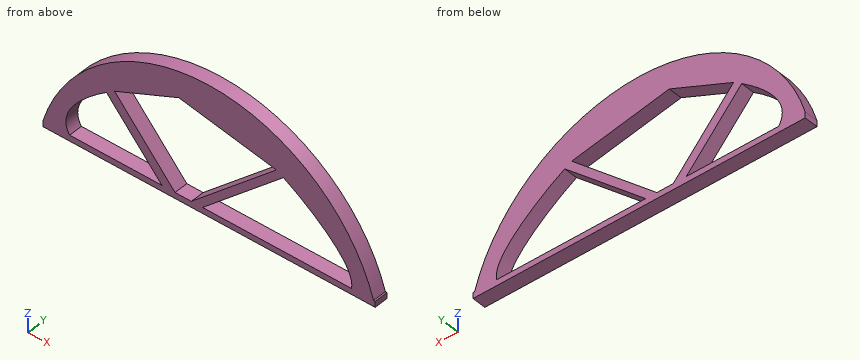
```python
from build123d import *

# Parameters (mm, degrees)
F1_DEPTH = 76.2


with BuildPart() as f1:
    # F0 (on Front) → F1 (new body)
    with BuildSketch(Plane.XZ):
        with BuildLine():
            Line((900.6498717056, -312.5507702395), (891.7103917568, -312.5507702395))
            ThreePointArc((891.7103917568, -312.5507702395), (-18.2198682688, 368.2339185386), (-928.1501282944, -312.5507702395))
            Line((-928.1501282944, -312.5507702395), (-928.1501282944, -345.05851352))
            Line((-928.1501282944, -345.05851352), (-749.2538985146, -345.05851352))
            add(Edge.make_bspline(
                [(-749.2538985146, -345.0585135201), (-760.7342074403, -336.2080146902), (-770.4190479747, -326.955384148), (-778.1336966335, -317.3006312947)],
                knots=[0.9863041687, 0.9863041687, 0.9863041687, 0.9863041687, 1, 1, 1, 1], degree=3))
            add(Edge.make_bspline(
                [(-778.1336966335, -317.3006312947), (-779.3903781429, -315.7279155528), (-780.5947807249, -314.1445295186), (-781.7476175602, -312.5507702395)],
                knots=[0, 0, 0, 0, 0.0022309892, 0.0022309892, 0.0022309892, 0.0022309892], degree=3))
            add(Edge.make_bspline(
                [(-781.7476175602, -312.5507702395), (-852.1024790666, -215.2874716318), (-730.4075461351, -79.390396257), (-578.7611195863, 27.6247892302)],
                knots=[0.0022309892, 0.0022309892, 0.0022309892, 0.0022309892, 0.1383828997, 0.1383828997, 0.1383828997, 0.1383828997], degree=3))
            add(Edge.make_bspline(
                [(-578.7611195863, 27.6247892302), (-564.0565616619, 38.0016311354), (-549.0703872563, 48.1069134214), (-533.9503839152, 57.8790810031)],
                knots=[0.1383828997, 0.1383828997, 0.1383828997, 0.1383828997, 0.1515850153, 0.1515850153, 0.1515850153, 0.1515850153], degree=3))
            add(Edge.make_bspline(
                [(-533.9503839241, 57.8790809984), (-602.4722852405, 100.7350307252), (-409.6251199582, 190.8667602879), (-180.120050854, 211.9691197295)],
                knots=[0, 0, 0, 0, 0.2694339971, 0.2694339971, 0.2694339971, 0.2694339971], degree=3))
            add(Edge.make_bspline(
                [(-180.1200508538, 211.9691197281), (-93.8173354063, 228.6015651353), (-14.6508277799, 226.1155115237), (65.4117966901, 211.4804253565)],
                knots=[0.2631178936, 0.2631178936, 0.2631178936, 0.2631178936, 0.3555862093, 0.3555862093, 0.3555862093, 0.3555862093], degree=3))
            add(Edge.make_bspline(
                [(65.4117966901, 211.4804253565), (252.144781627, 195.4027277771), (400.2346102312, 147.7404794914), (357.158674228, 108.3680934352)],
                knots=[0.3646274658, 0.3646274658, 0.3646274658, 0.3646274658, 0.5902554086, 0.5902554086, 0.5902554086, 0.5902554086], degree=3))
            add(Edge.make_bspline(
                [(357.1586742266, 108.3680934339), (369.9420280531, 101.672338017), (382.7382890401, 94.6802256262), (395.5442289819, 87.3893097061)],
                knots=[0.4659511905, 0.4659511905, 0.4659511905, 0.4659511905, 0.4802734469, 0.4802734469, 0.4802734469, 0.4802734469], degree=3))
            add(Edge.make_bspline(
                [(395.5442289819, 87.3893097061), (452.0964892557, 55.1919250067), (621.2097193886, -58.1382004272), (789.5300294959, -225.1035077486), (769.7574939756, -312.5507702395)],
                knots=[0.4802734469, 0.4802734469, 0.4802734469, 0.4802734469, 0.5435219059, 0.668781717, 0.668781717, 0.668781717, 0.668781717], degree=3))
            add(Edge.make_bspline(
                [(769.7574939756, -312.5507702395), (767.2117421615, -323.809772753), (762.4841536184, -334.6792525956), (755.294559917, -345.05851352)],
                knots=[0.668781717, 0.668781717, 0.668781717, 0.668781717, 0.6849091576, 0.6849091576, 0.6849091576, 0.6849091576], degree=3))
            Line((755.2945599171, -345.05851352), (900.6498717056, -345.05851352))
            Line((900.6498717056, -345.05851352), (900.6498717056, -312.5507702395))
        make_face()
        with BuildLine():
            add(Edge.make_bspline(
                [(-749.2538985146, -345.0585135201), (-760.7342074403, -336.2080146902), (-770.4190479747, -326.955384148), (-778.1336966335, -317.3006312947)],
                knots=[0.9863041687, 0.9863041687, 0.9863041687, 0.9863041687, 1, 1, 1, 1], degree=3))
            Line((-749.2538985146, -345.05851352), (755.2945599171, -345.05851352))
            add(Edge.make_bspline(
                [(769.7574939756, -312.5507702395), (767.2117421615, -323.809772753), (762.4841536184, -334.6792525956), (755.294559917, -345.05851352)],
                knots=[0.668781717, 0.668781717, 0.668781717, 0.668781717, 0.6849091576, 0.6849091576, 0.6849091576, 0.6849091576], degree=3))
            Line((769.7574939756, -312.5507702395), (-49.9293302995, -312.5507702395))
            Line((-49.9293302995, -312.5507702395), (395.5442289819, 87.3893097061))
            add(Edge.make_bspline(
                [(357.1586742266, 108.3680934339), (369.9420280531, 101.672338017), (382.7382890401, 94.6802256262), (395.5442289819, 87.3893097061)],
                knots=[0.4659511905, 0.4659511905, 0.4659511905, 0.4659511905, 0.4802734469, 0.4802734469, 0.4802734469, 0.4802734469], degree=3))
            add(Edge.make_bspline(
                [(357.158674228, 108.3680934352), (356.9910150595, 108.2148491387), (356.8204599128, 108.0617304257), (356.6470209458, 107.9087381034)],
                knots=[0.5902554086, 0.5902554086, 0.5902554086, 0.5902554086, 0.5911335925, 0.5911335925, 0.5911335925, 0.5911335925], degree=3))
            Line((356.6470209458, 107.9087381034), (-111.6821191112, -312.5507702395))
            Line((-111.6821191112, -312.5507702395), (-201.3835205481, -312.5507702395))
            Line((-201.3835205481, -312.5507702395), (-533.9503839109, 57.8790810059))
            add(Edge.make_bspline(
                [(-578.7611195863, 27.6247892302), (-564.0565616619, 38.0016311354), (-549.0703872563, 48.1069134214), (-533.9503839152, 57.8790810031)],
                knots=[0.1383828997, 0.1383828997, 0.1383828997, 0.1383828997, 0.1515850153, 0.1515850153, 0.1515850153, 0.1515850153], degree=3))
            Line((-578.7611195863, 27.6247892302), (-273.35614635, -312.5507702395))
            Line((-273.35614635, -312.5507702395), (-781.7476175602, -312.5507702395))
            add(Edge.make_bspline(
                [(-778.1336966335, -317.3006312947), (-779.3903781429, -315.7279155528), (-780.5947807249, -314.1445295186), (-781.7476175602, -312.5507702395)],
                knots=[0, 0, 0, 0, 0.0022309892, 0.0022309892, 0.0022309892, 0.0022309892], degree=3))
        make_face()
        with BuildLine():
            Line((-180.120050854, 211.9691197295), (357.1586742266, 108.3680934339))
            add(Edge.make_bspline(
                [(65.4117966901, 211.4804253565), (71.5175240267, 210.3643259746), (167.1573362354, 191.7908820713), (264.946329488, 156.6677270957), (357.1586742266, 108.3680934339)],
                knots=[0.3555862093, 0.3555862093, 0.3555862093, 0.3555862093, 0.3626380181, 0.4659511905, 0.4659511905, 0.4659511905, 0.4659511905], degree=3))
            add(Edge.make_bspline(
                [(-180.120050854, 211.9691197295), (-99.0338336855, 219.424774226), (-13.3717100026, 218.2636800411), (65.4117966901, 211.4804253565)],
                knots=[0.2694339971, 0.2694339971, 0.2694339971, 0.2694339971, 0.3646274658, 0.3646274658, 0.3646274658, 0.3646274658], degree=3))
        make_face()
        with BuildLine():
            add(Edge.make_bspline(
                [(65.4117966901, 211.4804253565), (71.5175240267, 210.3643259746), (167.1573362354, 191.7908820713), (264.946329488, 156.6677270957), (357.1586742266, 108.3680934339)],
                knots=[0.3555862093, 0.3555862093, 0.3555862093, 0.3555862093, 0.3626380181, 0.4659511905, 0.4659511905, 0.4659511905, 0.4659511905], degree=3))
            add(Edge.make_bspline(
                [(65.4117966901, 211.4804253565), (252.144781627, 195.4027277771), (400.2346102312, 147.7404794914), (357.158674228, 108.3680934352)],
                knots=[0.3646274658, 0.3646274658, 0.3646274658, 0.3646274658, 0.5902554086, 0.5902554086, 0.5902554086, 0.5902554086], degree=3))
        make_face()
        with BuildLine():
            add(Edge.make_bspline(
                [(-533.9503839241, 57.8790809984), (-602.4722852405, 100.7350307252), (-409.6251199582, 190.8667602879), (-180.120050854, 211.9691197295)],
                knots=[0, 0, 0, 0, 0.2694339971, 0.2694339971, 0.2694339971, 0.2694339971], degree=3))
            add(Edge.make_bspline(
                [(-533.9503839152, 57.8790810031), (-491.8326282353, 85.1000913023), (-360.9478670377, 159.8172978773), (-249.892894391, 198.5223468773), (-180.1200508538, 211.9691197281)],
                knots=[0.1515850153, 0.1515850153, 0.1515850153, 0.1515850153, 0.1883603696, 0.2631178936, 0.2631178936, 0.2631178936, 0.2631178936], degree=3))
        make_face()
        with BuildLine():
            add(Edge.make_bspline(
                [(-533.9503839152, 57.8790810031), (-491.8326282353, 85.1000913023), (-360.9478670377, 159.8172978773), (-249.892894391, 198.5223468773), (-180.1200508538, 211.9691197281)],
                knots=[0.1515850153, 0.1515850153, 0.1515850153, 0.1515850153, 0.1883603696, 0.2631178936, 0.2631178936, 0.2631178936, 0.2631178936], degree=3))
            Line((-533.9503839109, 57.8790810059), (-180.120050854, 211.9691197295))
        make_face()
        with BuildLine():
            add(Edge.make_bspline(
                [(-180.120050854, 211.9691197295), (-99.0338336855, 219.424774226), (-13.3717100026, 218.2636800411), (65.4117966901, 211.4804253565)],
                knots=[0.2694339971, 0.2694339971, 0.2694339971, 0.2694339971, 0.3646274658, 0.3646274658, 0.3646274658, 0.3646274658], degree=3))
            add(Edge.make_bspline(
                [(-180.1200508538, 211.9691197281), (-93.8173354063, 228.6015651353), (-14.6508277799, 226.1155115237), (65.4117966901, 211.4804253565)],
                knots=[0.2631178936, 0.2631178936, 0.2631178936, 0.2631178936, 0.3555862093, 0.3555862093, 0.3555862093, 0.3555862093], degree=3))
        make_face()
    extrude(amount=F1_DEPTH)


solid = f1.part
```
CAD build for the part. Positions are in the model's coordinates, mm. Give positions to 0.01 mm unless a question says otherwise; leave off trailing zeros. Order: outer loops, then holes, each group sorted by start corner. A loop starts at its lowest first (then second) coordinate and runs counter-clockwise, first axis right, second up.
(1) Saw through at D-D, the plane x = 303. Give the cut face in (y, z).
(2) Saw through at C-C, the plane y = -63.5. State how many separate pieces and enclosed holes the cut face has, then the cut area to 3 significant figures.
(3) Flat gauge pins, fed straight in: pin 1 (6 mm diameter, centred on x = 578.5, z = 14, fed in from +Y); pin 2 (10 mm diameter, centred on x = 618, y = -57, fed in from +Z); pin 3 (23 mm diameter, centred on x = 287, y = -37.5, fed in from +Z); pin 4 (23 mm diameter, centred on x = -528.5, y = -54.5, fed in from +Z). Where does each tip first touch, or does it go through?
(4) Saw through at A-A, the plane x = -137.5. Give the cut face in (y, z).
(5) Drill centre lines: L1, parallel to X at y = -35.5, z = -307.5; L2, parallel to X at y = -21, z = -201.5; L3, parallel to Z at x = -432.5, y = -17. Where is each one in solid material? Low to high.
(6) Saw through at B-B, the plane z = 171. Give the cut face in (x, y).
Results found:
1. outline: (-76.2, -345.06) - (0, -345.06) - (0, -312.55) - (-76.2, -312.55) - close; (-76.2, 4.3) - (0, 4.3) - (0, 59.75) - (-76.2, 59.75) - close; (-76.2, 118.81) - (0, 118.81) - (0, 312.19) - (-76.2, 312.19) - close
2. separate pieces: 1
2. enclosed holes: 3
2. area: 428,000 mm2
3. pin 1: stops at y = 0
3. pin 2: stops at z = 127.7
3. pin 3: stops at z = 321.61
3. pin 4: stops at z = 226.5
4. outline: (-76.2, -345.06) - (0, -345.06) - (0, -312.55) - (-76.2, -312.55) - close; (-76.2, 203.75) - (0, 203.75) - (0, 360.7) - (-76.2, 360.7) - close
5. L1: x = -926.65 to -785.21, -277.89 to -205.92, -106.06 to -44.3, 770.75 to 890.21
5. L2: x = -887.81 to -792.88, -373.06 to -301.08, 12.01 to 73.76, 740.1 to 851.37
5. L3: z = -345.06 to -312.55, -135.29 to -55.12, 102.06 to 272.98
6. outline: (-597.23, -76.2) - (-274.2, -76.2) - (-274.2, 0) - (-597.23, 0) - close; (32.35, -76.2) - (560.79, -76.2) - (560.79, 0) - (32.35, 0) - close
